The listing builds one solid part. Answer for the finished solid, in the listing's coordinates (mm). Face numbers are marked on the shaded views. A direction names the side the tool comes from. Give positions to 0.01 mm unless a question says otherwise; leave off trailing zeros. Order: outer loops, then holes, each group sorted by start corner. A loop starts at its lowest first (then second) coordinate and runs counter-clockwise, first axis right, second up. Notation, with made-up numbers: (58.5, -23) - (68.5, -23) arc R16 ccw to (68.5, -10) - close; hole circle Ø4 at (-31.5, 26). An arc over 180 degrees is marked (long way). Answer in a Markdown table with one row per item.
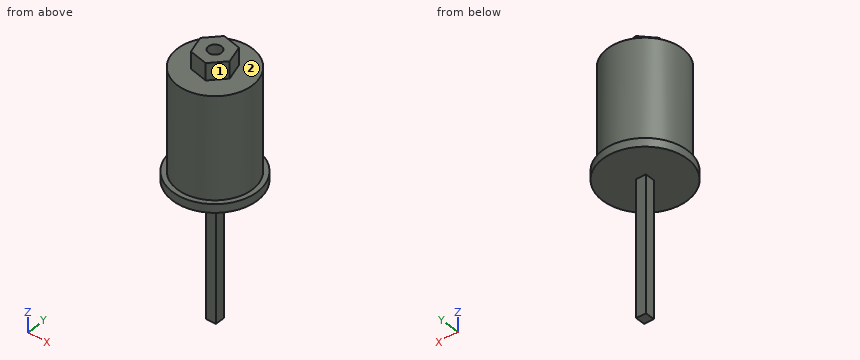
Autodesk Inventor part; units mm, degrees
ref_plane "YZ Plane" through (0, 0, 0) normal (1, 0, 0) x (0, 1, 0)
ref_plane "XZ Plane" through (0, 0, 0) normal (0, 1, 0) x (-1, 0, 0)
ref_plane "XY Plane" through (0, 0, 0) normal (0, 0, 1) x (1, 0, 0)
sketch "Sketch1" plane through (0, 0, 0) normal (0, 0, 1) x (1, 0, 0)
  circle A0 centre (0, 0) radius 15.875
  dimension "d0" = 31.75
extrude "Extrusion1" add sketch "Sketch1" along normal blind 3.175
sketch "Sketch2" plane through (0, 0, 3.175) normal (0, 0, 1) x (1, 0, 0)
  circle A0 centre (0, 0) radius 14.0335
  dimension "d3" = 28.067
extrude "Extrusion2" add sketch "Sketch2" along normal blind 38.1
sketch "Sketch3" plane through (0, 0, 41.275) normal (0, 0, 1) x (1, 0, 0)
  line L0 (6.851, -1.6161) -> (2.0259, -6.7412)
  line L1 (2.0259, -6.7412) -> (-4.8251, -5.1251)
  line L2 (-4.8251, -5.1251) -> (-6.851, 1.6161)
  line L3 (-6.851, 1.6161) -> (-2.0259, 6.7412)
  line L4 (-2.0259, 6.7412) -> (4.8251, 5.1251)
  line L5 (4.8251, 5.1251) -> (6.851, -1.6161)
  point P0 (0, 0)
  point P1 (0, 0)
  dimension "d6" = 12.192
extrude "Extrusion3" add sketch "Sketch3" along normal blind 6.35
sketch "Sketch4" plane through (0, 0, 47.625) normal (0, 0, 1) x (1, 0, 0)
  circle A0 centre (0, 0) radius 2.4511
  dimension "d9" = 4.9022
extrude "Extrusion4" cut sketch "Sketch4" against normal blind 19.05
sketch "Sketch5" plane through (0, 0, 0) normal (0, 0, -1) x (-1, 0, 0)
  line L0 (1.8415, 1.8415) -> (-1.8415, 1.8415)
  line L1 (-1.8415, 1.8415) -> (-1.8415, -1.8415)
  line L2 (-1.8415, -1.8415) -> (1.8415, -1.8415)
  line L3 (1.8415, -1.8415) -> (1.8415, 1.8415)
  point P0 (0, 0)
  point P1 (0, -1.8415)
  point P2 (1.8415, 0)
  dimension "d12" = 3.683
extrude "Extrusion5" add sketch "Sketch5" along normal blind 50.8
sketch "Sketch6" plane through (0, 0, 0) normal (0, 0, -1) x (-1, 0, 0)
  point P0 (0, 0)
properties part number "drive shaft"
Item 1: Each of these flat-tipped pins is pushed along its axis until it touches: P1, Ø3, axis at x = -9.5, y = -0.5, coming from the +Z side (3 decimals); P2, Ø5, axis at y = 4.5, z = 28.5, coming from the +X side; P3, Ø1.1, axis at x = 0.5, z = -35.5, coming from the +Y side. Where does it stop, or does it pass through?
Answer block:
| item | result |
|---|---|
| P1 | z = 41.275 |
| P2 | x = 13.89 |
| P3 | y = 1.84 |
Item 2: Find section C-C on z = 38. Write down the section's boundary in (x, y), then the cut area to 3 significant figures.
Answer block:
| item | result |
|---|---|
| outline | circle Ø28.07 at (0, 0); hole circle Ø4.9 at (0, 0) |
| area | 600 mm² |
Item 3: Find section D-D on z = 26. Write down the section's boundary in (x, y).
Answer block:
| item | result |
|---|---|
| outline | circle Ø28.07 at (0, 0) |
Item 4: Find section B-B on y = 0. Write down the section's boundary in (x, z) (1 decimal).
Answer block:
| item | result |
|---|---|
| outline | (-15.9, 0) - (-1.8, 0) - (-1.8, -50.8) - (1.8, -50.8) - (1.8, 0) - (15.9, 0) - (15.9, 3.2) - (14, 3.2) - (14, 41.3) - (6.4, 41.3) - (6.4, 47.6) - (2.5, 47.6) - (2.5, 28.6) - (-2.5, 28.6) - (-2.5, 47.6) - (-6.4, 47.6) - (-6.4, 41.3) - (-14, 41.3) - (-14, 3.2) - (-15.9, 3.2) - close |
Item 5: Find section A-A on x = 8. Write down the section's boundary in (y, z) (3 decimals), then the cut area to 3 significant figures.
Answer block:
| item | result |
|---|---|
| outline | (-13.712, 0) - (13.712, 0) - (13.712, 3.175) - (11.53, 3.175) - (11.53, 41.275) - (-11.53, 41.275) - (-11.53, 3.175) - (-13.712, 3.175) - close |
| area | 966 mm² |
Item 6: Which of the six approach directions +Z, -Z, +X, -X, +Y, -Y give full straight-line access (tool end or side, diameter ignored) to the marked faces 1 and 2?
Answer block:
| item | result |
|---|---|
| face 1 | +Z, +X, -Y |
| face 2 | +Z |
Item 7: Consider line 1 (Y direction, x = 0, z = 39); line 2 (Z direction, x = -7.5, y = -5) (3 decimals); line 3 (Z direction, x = -4.5, y = -14) (3 decimals). Determine where each line is inside the solid, lowest interval first.
Answer block:
| item | result |
|---|---|
| line 1 | -14.03 to -2.45, 2.45 to 14.03 |
| line 2 | 0 to 41.275 |
| line 3 | 0 to 3.175 |
